CAD build for the part. Positions are in the model's coordinates, mm. A direction names the side the tool comes from. Give positions to 0.01 mm unless a question says otherwise; leave off trailing zeros. Loops run counter-clockwise (first coordinate to the right, second up) from the corner with the lowest first, then second, coordinate; pieces in that order, holes last. Notation, with made-up numbers: (-6, -2.75) -> (12, -2.75) arc R21 cw to (12, 23.25) -> close; hole circle Ø9 at (39, 19). An arc over 180 degrees is marked (long way). Use one line per item in the form item = value.
```python
from build123d import *

# Parameters (mm, degrees)
F0_R     = 19.05
F1_DEPTH = 50.8
F2_DEPTH = 44.45
F0_R_2   = 9.525
F3_DEPTH = 44.45
F5_DEPTH = 6.35


with BuildPart() as f1:
    # F0 (on Right) → F1 (new body)
    with BuildSketch(Plane.YZ):
        with BuildLine():
            ThreePointArc((-24.8587950459, 5.2153915354), (-2.6216984795, -25.2643364663), (25.4, 0))
            ThreePointArc((25.4, 0), (25.2643364465, 2.6216986701), (24.8587949672, 5.2153919105))
            ThreePointArc((24.8587949672, 5.2153919105), (-1.916e-07, 25.4), (-24.8587950459, 5.2153915354))
        make_face()
        Circle(F0_R, mode=Mode.SUBTRACT)
    extrude(amount=F1_DEPTH)

    # F0 (on Right) → F2 (join)
    with BuildSketch(Plane.YZ):
        with BuildLine():
            ThreePointArc((-24.8587950459, 5.2153915354), (-1.916e-07, 25.4), (24.8587949672, 5.2153919105))
            Line((24.8587949672, 5.2153919105), (12.7, 63.1694245347))
            ThreePointArc((12.7, 63.1694245347), (0, 50.4694245347), (-12.7, 63.1694245347))
            Line((-12.7, 63.1694245347), (-24.8587950459, 5.2153915354))
        make_face()
    extrude(amount=F2_DEPTH)

    # F0 (on Right) → F3 (join)
    with BuildSketch(Plane.YZ):
        with BuildLine():
            ThreePointArc((-12.7, 63.1694245347), (0, 50.4694245347), (12.7, 63.1694245347))
            ThreePointArc((12.7, 63.1694245347), (0, 75.8694245347), (-12.7, 63.1694245347))
        make_face()
        with Locations((0, 63.1694245347)):
            Circle(F0_R_2, mode=Mode.SUBTRACT)
    extrude(amount=F3_DEPTH)

    # F4 (on face) → F5 (cut)
    with BuildSketch(Plane.YZ.offset(44.45)):
        with BuildLine():
            ThreePointArc((-23.7782567625, 8.9305377965), (1.9345459415, 25.3262222212), (24.8587949734, 5.2153918809))
            Line((24.8587949672, 5.2153919105), (12.7, 63.1694245347))
            ThreePointArc((12.7, 63.1694245347), (0, 47.5284621589), (-12.7, 63.1694245347))
            Line((-12.7, 63.1694245347), (-24.8587950459, 5.2153915354))
            ThreePointArc((-24.8587950459, 5.2153915354), (-24.3893681773, 7.0935689122), (-23.7782567625, 8.9305377965))
        make_face()
    extrude(amount=-F5_DEPTH, mode=Mode.SUBTRACT)


solid = f1.part
```
1. Cut at C-C, the plane z = -2. Write the cut outline in (x, y), then the cut area to 3 significant figures.
Result sheet:
outline = (0, -25.32) -> (50.8, -25.32) -> (50.8, -18.94) -> (0, -18.94) -> close; (0, 18.94) -> (50.8, 18.94) -> (50.8, 25.32) -> (0, 25.32) -> close
area = 648 mm^2
2. Cut at D-D, the plane y = 15. Write the cut outline in (x, z).
Result sheet:
outline = (0, -20.5) -> (50.8, -20.5) -> (50.8, -11.74) -> (0, -11.74) -> close; (0, 11.74) -> (50.8, 11.74) -> (50.8, 20.5) -> (38.1, 20.5) -> (38.1, 52.21) -> (0, 52.21) -> close
3. Mould opens along Y. For faces 1 (the cylindrical face through (25.04, -15.12, -11.59)), 2 (the flat face through (18.783, 18.865, 33.787)), 3 (the cylindrical face through (41.319, 0.323, 47.532)), 4 (the flat face through (18.783, -18.694, 34.598)) say: pulls with the +Y half, pulls with the -Y half, needs draft (parallel to the pull), parting line crosses it, or undercut.
Result sheet:
face_1 = undercut
face_2 = pulls with the +Y half
face_3 = parting line crosses it
face_4 = pulls with the -Y half
4. Drop flat-ended pins along their axis: P1, Ø1.5, axis at x = 35, y = 18.5, coming from the -Z side; P2, Ø5, axis at x = 33.5, z = 14.5, coming from the +Y side; P3, Ø8, axis at x = 11.5, z = 11.5, coming from the -Y side; P4, Ø6, axis at y = 19, z = 7.5, coming from the -X side. Give the stop position or say it passes through.
Result sheet:
P1 = -18.17
P2 = 23.44
P3 = -24.38
P4 = 0
5. Cut at B-B, the plane y = 0. Write the cut outline in (x, z).
Result sheet:
outline = (0, -25.4) -> (50.8, -25.4) -> (50.8, -19.05) -> (0, -19.05) -> close; (0, 19.05) -> (50.8, 19.05) -> (50.8, 25.4) -> (38.1, 25.4) -> (38.1, 47.53) -> (44.45, 47.53) -> (44.45, 53.64) -> (0, 53.64) -> close; (0, 72.69) -> (44.45, 72.69) -> (44.45, 75.87) -> (0, 75.87) -> close
6. Tool access for faces 5 (the flat face through (44.45, 0, 52)), 6 (the cylindrical face through (21.91, -2.06, 53.87)): list every direction of +Z, -Z, +X, -X, +Y, -Y with a clear straight run to the whole face (end or side of a thin tool).
Result sheet:
face_5 = +Z, +X, +Y, -Y
face_6 = +X, -X
7. Drill centre lines: line 1 (Z direction, x = 32, y = 0); line 2 (Z direction, x = 16.5, y = 4); line 3 (X direction, y = -21, z = 17.5). Where is each one in solid material? Low to high.
Result sheet:
line_1 = -25.4 to -19.05, 19.05 to 53.64, 72.69 to 75.87
line_2 = -25.08 to -18.63, 18.63 to 54.53, 71.81 to 75.22
line_3 = 0 to 38.1
8. Cut at A-A, the plane x = 26. Write the cut outline in (y, z) (3 decimals), then the cut area to 3 significant figures.
Result sheet:
outline = (-24.859, 5.215) arc R25.4 ccw (long way) to (24.859, 5.215) -> (12.7, 63.169) arc R12.7 ccw to (-12.7, 63.169) -> close; hole circle Ø38.1 at (0, 0); hole circle Ø19.05 at (0, 63.169)
area = 2,280 mm^2
